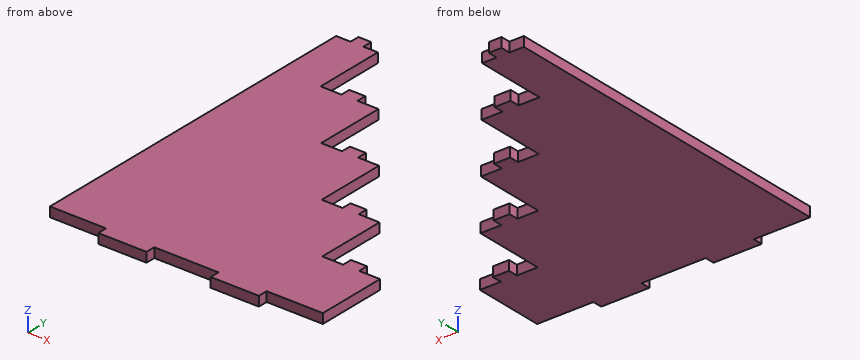
```python
from build123d import *

# Parameters (mm, degrees)
BOSS_EXTRU_1_DEPTH = 6
ESQUISSE2_W        = 30
ESQUISSE2_H        = 6
BOSS_EXTRU_2_DEPTH = 6
ESQUISSE3_W        = 8
ESQUISSE3_H        = 6
BOSS_EXTRU_3_DEPTH = 6
ESQUISSE4_W        = 10
ESQUISSE4_H        = 6
BOSS_EXTRU_4_DEPTH = 6
ESQUISSE5_W        = 10
ESQUISSE5_H        = 6
BOSS_EXTRU_5_DEPTH = 6
ESQUISSE6_W        = 10
ESQUISSE6_H        = 6
BOSS_EXTRU_6_DEPTH = 6
ESQUISSE7_W        = 10
ESQUISSE7_H        = 6
BOSS_EXTRU_7_DEPTH = 6


with BuildPart() as part:
    # Esquisse1 → Boss.-Extru.1 (new body)
    with BuildSketch(Plane.XY):
        Polygon((0, 220), (26, 220), (26, 176), (62, 176), (62, 132), (98, 132), (98, 88), (134, 88), (134, 44), (170, 44), (170, 0), (0, 0), align=None)
    extrude(amount=BOSS_EXTRU_1_DEPTH)

    # Esquisse2 → Boss.-Extru.2 (add)
    with BuildSketch(Plane.XZ):
        with Locations((50, 3)):
            Rectangle(ESQUISSE2_W, ESQUISSE2_H)
        with Locations((120, 3)):
            Rectangle(ESQUISSE2_W, ESQUISSE2_H)
    extrude(amount=BOSS_EXTRU_2_DEPTH)

    # Esquisse3 → Boss.-Extru.3 (add)
    with BuildSketch(Plane(origin=(0, 220, 0), x_dir=(1, 0, 0), z_dir=(0, 1, 0))):
        with Locations((13, -3)):
            Rectangle(ESQUISSE3_W, ESQUISSE3_H)
    extrude(amount=BOSS_EXTRU_3_DEPTH)

    # Esquisse4 → Boss.-Extru.4 (add)
    with BuildSketch(Plane(origin=(0, 176, 0), x_dir=(1, 0, 0), z_dir=(0, 1, 0))):
        with Locations((44, -3)):
            Rectangle(ESQUISSE4_W, ESQUISSE4_H)
    extrude(amount=BOSS_EXTRU_4_DEPTH)

    # Esquisse5 → Boss.-Extru.5 (add)
    with BuildSketch(Plane(origin=(0, 132, 0), x_dir=(1, 0, 0), z_dir=(0, 1, 0))):
        with Locations((80, -3)):
            Rectangle(ESQUISSE5_W, ESQUISSE5_H)
    extrude(amount=BOSS_EXTRU_5_DEPTH)

    # Esquisse6 → Boss.-Extru.6 (add)
    with BuildSketch(Plane(origin=(0, 88, 0), x_dir=(1, 0, 0), z_dir=(0, 1, 0))):
        with Locations((116, -3)):
            Rectangle(ESQUISSE6_W, ESQUISSE6_H)
    extrude(amount=BOSS_EXTRU_6_DEPTH)

    # Esquisse7 → Boss.-Extru.7 (add)
    with BuildSketch(Plane(origin=(0, 44, 0), x_dir=(1, 0, 0), z_dir=(0, 1, 0))):
        with Locations((152, -3)):
            Rectangle(ESQUISSE7_W, ESQUISSE7_H)
    extrude(amount=BOSS_EXTRU_7_DEPTH)


solid = part.part
```
Here's how the part is built. I have some questions about the finished solid (model axes, mm). Give positions to 0.01 mm unless a question says otherwise; leave off trailing zeros. Order: outer loops, then holes, each group sorted by start corner. A loop starts at its lowest first (then second) coordinate and runs counter-clockwise, first axis right, second up. Notation, with made-up numbers: (16, 66) -> (71, 66) arc R20 ccw to (71, 100) -> close; hole circle Ø2 at (42.5, -26). An arc over 180 degrees is marked (long way). Use CSV: the item, a comma, the result in double quotes. Start each with the question number.
Item 1: I'm going to push flat-ended pins straight in: P1, Ø3, axis at y = -2, z = 4, coming from the -X side; P2, Ø1.8, axis at x = 152, z = 2.5, coming from the +Y side; P3, Ø3, axis at x = 55, z = 2, coming from the +Y side. Where does each tip first touch, or does it pass through?
Item 2: Suppose I cut it at B-B (x = 138.5). List the corners of the cut face in (y, z) for me.
Item 3: Suppose I cut it at A-A (y = 71.5). List the corners of the cut face in (x, z) for me, and give its area (3 significant figures).
Item 4: If I drill on probe 1 along X at (y, z) = (112.5, 0.45); probe 2 along X at (y, z) = (46.5, 3.8); probe 3 along Y at (x, z) = (59, 4.5), over which ranges is the centre line in solid material (lowest first)? Write a range as [from, to].
Answer block:
1,P1,"stops at x = 35"
1,P2,"stops at y = 50"
1,P3,"stops at y = 176"
2,outline,"(0, 0) -> (44, 0) -> (44, 6) -> (0, 6) -> close"
3,outline,"(0, 0) -> (134, 0) -> (134, 6) -> (0, 6) -> close"
3,area,"804 mm^2"
4,probe 1,"x = [0, 98]"
4,probe 2,"x = [0, 134], [147, 157]"
4,probe 3,"y = [-6, 176]"
